from build123d import *

# Parameters (mm, degrees)
ESQUISSE1_R             = 19.25
BOSS_EXTRU_1_DEPTH      = 13
BOSS_EXTRU_1_DEPTH_BACK = 27
ESQUISSE1_6_R           = 4.5
ESQUISSE1_6_R_2         = 19.25
BOSS_EXTRU_2_DEPTH      = 5
CHANFREIN1_SIZE         = 1
ESQUISSE6_R             = 9.9
BOSS_EXTRU_4_DEPTH      = 51
CHANFREIN2_SIZE         = 6
CHANFREIN2_SIZE2        = 12.867041523


with BuildPart() as part:
    # Esquisse1 → Boss.-Extru.1 (new body, two sides)
    with BuildSketch(Plane.XY) as boss_extru_1_sk:
        Circle(ESQUISSE1_R)
    extrude(amount=BOSS_EXTRU_1_DEPTH)
    extrude(boss_extru_1_sk.sketch, amount=-BOSS_EXTRU_1_DEPTH_BACK)

    # Esquisse1_6 → Boss.-Extru.2 (add)
    with BuildSketch(Plane.XY):
        with BuildLine():
            Line((34.228492936, 28), (0, 28))
            Line((0, 28), (-34.228492936, 28))
            ThreePointArc((-34.228492936, 28), (-37.239470502, 26.991743241), (-39.036112674, 24.373605639))
            Line((-39.036112674, 24.373605639), (-45.347302875, 2.284439938))
            ThreePointArc((-45.347302875, 2.284439938), (-45.721922521, -0.012532828), (-45.555449063, -2.33389242))
            Line((-45.555449063, -2.33389242), (-38.774178945, -37.935560539))
            ThreePointArc((-38.774178945, -37.935560539), (-37.050133937, -40.852129456), (-33.862486113, -42))
            Line((-33.862486113, -42), (33.862486113, -42))
            ThreePointArc((33.862486113, -42), (37.050133937, -40.852129456), (38.774178945, -37.935560539))
            Line((38.774178945, -37.935560539), (45.555449063, -2.33389242))
            ThreePointArc((45.555449063, -2.33389242), (45.721922521, -0.012532828), (45.347302875, 2.284439938))
            Line((45.347302875, 2.284439938), (39.036112674, 24.373605639))
            ThreePointArc((39.036112674, 24.373605639), (37.239470502, 26.991743241), (34.228492936, 28))
        make_face()
        with Locations((-30, -32)):
            Circle(ESQUISSE1_6_R, mode=Mode.SUBTRACT)
        with Locations((30, -32)):
            Circle(ESQUISSE1_6_R, mode=Mode.SUBTRACT)
        with Locations((-35, 0)):
            Circle(ESQUISSE1_6_R, mode=Mode.SUBTRACT)
        Circle(ESQUISSE1_6_R_2, mode=Mode.SUBTRACT)
        with Locations((-30, 18)):
            Circle(ESQUISSE1_6_R, mode=Mode.SUBTRACT)
        with Locations((35, 0)):
            Circle(ESQUISSE1_6_R, mode=Mode.SUBTRACT)
        with Locations((30, 18)):
            Circle(ESQUISSE1_6_R, mode=Mode.SUBTRACT)
    extrude(amount=-BOSS_EXTRU_2_DEPTH)

    # Chanfrein1
    chanfrein1_edges = [part.edges().sort_by_distance(p)[0] for p in [
        (-19.25, 0, 13),
    ]]
    chamfer(chanfrein1_edges, length=CHANFREIN1_SIZE)

    # Esquisse6 → Boss.-Extru.4 (add)
    with BuildSketch(Plane(origin=(0, 0, -27), x_dir=(-1, 0, 0), z_dir=(0, 0, -1))):
        with Locations(Location((0, 0, 0), (0, 0, 180))):  # turned: the seam where the file's is
            Circle(ESQUISSE6_R)
    extrude(amount=BOSS_EXTRU_4_DEPTH)

    # Chanfrein2
    chanfrein2_edges = [part.edges().sort_by_distance(p)[0] for p in [
        (-19.25, 0, -27),
    ]]
    chanfrein2_side = [part.faces().sort_by_distance(p)[0] for p in [
        (-18.705527778, 0, -27),
    ]]
    chamfer(chanfrein2_edges, length=CHANFREIN2_SIZE, length2=CHANFREIN2_SIZE2, reference=chanfrein2_side[0])


solid = part.part
The model under review builds one solid part; all positions refer to its coordinate system, in mm. A direction names the side the tool comes from. Give positions to 0.01 mm unless a question says otherwise; leave off trailing zeros. Loops run counter-clockwise (first coordinate to the right, second up) from the corner with the lowest first, then second, coordinate; pieces in that order, holes last. Notation, with made-up numbers: (80, 5) -> (88, 5) arc R11 cw to (88, 15) -> close; hole circle Ø11 at (73.5, 49). An arc over 180 degrees is marked (long way). Answer as a JSON object with one key per item and string values. Group by question number.
Q1. Draft analysis for pull direction Y (two halves, no side actions). For faces 4 (the cylindrical face through (39.292, 1.352, -2.465)), 5 (the flat face through (-1, -22, -5)), 6 (the cylindrical face through (9.443, -2.974, -52.143)), state which applies: pulls with the +Y half, pulls with the -Y half, needs draft (parallel to the pull), parting line crosses it, or undercut.
Q2. Wall thickness on line 1 along Y through (x, z) = (-30, -2.6); line 2 along Z through (x, y) = (-11.5, -21); line 3 along Y through (x, z) = (35, -2): over which ranges is each line inside the solid? List them lowest first.
Q3. Tool access review of faces 1 (the cylindrical face through (-15.28, -11.71, 6.08)), 2 (the cylindrical face through (37.013, -40.883, -2.465)), 3 (the flat face through (-5, -9, -27)): name each direction out of +Z, -Z, +X, -X, +Y, -Y from which nothing blocks a thin tool from reaching the whole face with its end or side.
Q4. Take a section at D-D (y = 0). Write out the cut boundary in (x, z).
Q5. Insertion check: pin 1 (14.5 mm diameter, centred on x = 30, y = -32, fed in from +Z); pin 2 (6 mm diameter, centred on x = 2, z = -40, fed in from +Y); pin 3 (8 mm diameter, centred on x = -16, y = 16, fed in from -Z); pin 4 (7 mm diameter, centred on x = -30, y = 18, fed in from +Z). Each pin has a flat end and moves straight along its axis. Give the tip position at first contact, or say it passes through.
Q6. Take a section at B-B (x = 0). Write out the cut boundary in (y, z).
Q7. Take a section at A-A (y = -32). Write out the cut boundary in (x, z).
Q8. Take a section at C-C (z = -58.5). Write out the cut boundary in (x, y), plus the area to 3 significant figures.
Answer below:
{
 "1": {"face 4": "undercut", "face 5": "needs draft", "face 6": "parting line crosses it"},
 "2": {"line 1": "y = -42 to -36.5, -27.5 to 13.5, 22.5 to 28", "line 2": "z = -5 to 0", "line 3": "y = -41.87 to -4.5, 4.5 to 27.94"},
 "3": {"face 1": "+Z", "face 2": "+Z, -Z, +X, -Y", "face 3": "-Z"},
 "4": {"outline": "(-45.72, -5) -> (-39.5, -5) -> (-39.5, 0) -> (-45.72, 0) -> close; (-30.5, -5) -> (-19.25, -5) -> (-19.25, -14.13) -> (-13.25, -27) -> (-9.9, -27) -> (-9.9, -78) -> (9.9, -78) -> (9.9, -27) -> (13.25, -27) -> (19.25, -14.13) -> (19.25, -5) -> (30.5, -5) -> (30.5, 0) -> (19.25, 0) -> (19.25, 12) -> (18.25, 13) -> (-18.25, 13) -> (-19.25, 12) -> (-19.25, 0) -> (-30.5, 0) -> close; (39.5, -5) -> (45.72, -5) -> (45.72, 0) -> (39.5, 0) -> close"},
 "5": {"pin 1": "stops at z = 0", "pin 2": "stops at y = 9.9", "pin 3": "stops at z = -15.47", "pin 4": "passes through"},
 "6": {"outline": "(-42, -5) -> (-19.25, -5) -> (-19.25, -14.13) -> (-13.25, -27) -> (-9.9, -27) -> (-9.9, -78) -> (9.9, -78) -> (9.9, -27) -> (13.25, -27) -> (19.25, -14.13) -> (19.25, -5) -> (28, -5) -> (28, 0) -> (19.25, 0) -> (19.25, 12) -> (18.25, 13) -> (-18.25, 13) -> (-19.25, 12) -> (-19.25, 0) -> (-42, 0) -> close"},
 "7": {"outline": "(-39.9, -5) -> (-34.5, -5) -> (-34.5, 0) -> (-39.9, 0) -> close; (-25.5, -5) -> (25.5, -5) -> (25.5, 0) -> (-25.5, 0) -> close; (34.5, -5) -> (39.9, -5) -> (39.9, 0) -> (34.5, 0) -> close"},
 "8": {"outline": "circle Ø19.8 at (0, 0)", "area": "308 mm2"}
}
